from build123d import *

# Parameters (mm, degrees)
F0_W      = 50.8
F0_H      = 50.8
F0_W_2    = 39.37
F0_H_2    = 39.37
F1_DEPTH  = 25.4
F2_R      = 6.985
F3_DEPTH  = 50.801
F4_W      = 88.9
F4_H      = 279.4
F4_W_2    = 39.37
F4_H_2    = 39.37
F5_DEPTH  = 25.4
F6_W      = 76.2
F6_H      = 101.6
F7_DEPTH  = 3.175
F8_W      = 69.85
F8_H      = 101.6
F9_DEPTH  = 17.145
F10_W     = 69.85
F10_H     = 101.6
F11_DEPTH = 17.145
F12_W     = 38.1
F12_H     = 3.175
F13_DEPTH = 69.851
F15_DEPTH = 88.9


with BuildPart() as f1:
    # F0 (on Top) → F1 (new body)
    with BuildSketch(Plane.XY):
        Rectangle(F0_W, F0_H)
        Rectangle(F0_W_2, F0_H_2, mode=Mode.SUBTRACT)
    extrude(amount=F1_DEPTH)

    # F2 (on face) → F3 (cut, through all)
    with BuildSketch(Plane.XZ.offset(25.4)):
        with Locations((0, 12.7)):
            Circle(F2_R)
    extrude(amount=-F3_DEPTH, mode=Mode.SUBTRACT)

    # F4 (on face) → F5 (join)
    with BuildSketch(Plane.XY.offset(25.4)):
        Rectangle(F4_W, F4_H)
        Rectangle(F4_W_2, F4_H_2, mode=Mode.SUBTRACT)
    extrude(amount=F5_DEPTH)

    # F6 (on face) → F7 (cut)
    with BuildSketch(Plane(origin=(0, 0, 25.4), x_dir=(1, 0, 0), z_dir=(0, 0, -1))):
        with Locations((0, -82.55)):
            Rectangle(F6_W, F6_H)
        with Locations((0, 82.55)):
            Rectangle(F6_W, F6_H)
    extrude(amount=-F7_DEPTH, mode=Mode.SUBTRACT)

    # F8 (on face) → F9 (cut)
    with BuildSketch(Plane(origin=(0, 0, 28.575), x_dir=(1, 0, 0), z_dir=(0, 0, -1))):
        with Locations((0, -82.55)):
            Rectangle(F8_W, F8_H)
    extrude(amount=-F9_DEPTH, mode=Mode.SUBTRACT)

    # F10 (on face) → F11 (cut)
    with BuildSketch(Plane(origin=(0, 0, 28.575), x_dir=(1, 0, 0), z_dir=(0, 0, -1))):
        with Locations((0, 82.55)):
            Rectangle(F10_W, F10_H)
    extrude(amount=-F11_DEPTH, mode=Mode.SUBTRACT)

    # F12 (on face) → F13 (cut, through all)
    with BuildSketch(Plane.YZ.offset(25.4)):
        with Locations((0, 1.5875)):
            Rectangle(F12_W, F12_H)
    extrude(amount=-F13_DEPTH, mode=Mode.SUBTRACT)

    # F14 (on face) → F15 (join, through all)
    with BuildSketch(Plane.YZ.offset(44.45)):
        Polygon((-139.7, 25.4), (-139.7, 50.8), (-165.1, 50.8), align=None)
        Polygon((139.7, 50.8), (139.7, 25.4), (165.1, 50.8), align=None)
    extrude(amount=-F15_DEPTH)


solid = f1.part
Source: CAD feature listing. Evaluate the final solid. Frame: model axes, mm. A direction names the side the tool comes from. Round coordinates to 2 decimals unless told otherwise and drop trailing zeros. Write each loop counter-clockwise with the first axis right and the second up, starting at its lowest first coordinate (ties: lowest second). Pieces come first, ordered by that corner, then holes. Notation, with made-up numbers: M 77.25,53 L 134.25,53 A35 cw 134.25,85 Z; hole C -37.75,74.5 d7. An arc over 180 degrees is marked long. One line per item, written item: value. Start each with the question number.
Item 1: Section query D-D (x = 15.5). Return the cut outline in (y, z) (3 decimals).
Item 2: Set-up query: faces 4 (the flat face through (5, 25.4, 18)), 5 (the flat face through (-1, -31.75, 35)), 6 (the flat face through (25.4, 0, 13)), 7 (the flat face through (-19.685, 0, 31)), 8 (the flat face through (-44.45, -2, 38)). Return all of +Z, -Z, +X, -X, +Y, -Y with unobstructed straight access to the full face (end or side cutting, diameter ignored); none if empty.
Item 3: Ray query, L1, parallel to Y at x = -19, z = 7.5 (3 decimals); L2, parallel to Z at x = 0, y = -23.05 (3 decimals); L3, parallel to X at y = 22, z = 12. Return the intervals inside material, ascending. Write a range as from..to.
Item 4: Section query B-B (z = 12.7). Return the cut outline in (x, y) (3 decimals), plus the area to 3 significant figures.
Item 5: Mould query, pull axis Y, two halves, no side actions, for faces 1 (the flat face through (0.6, 152.2, 37.9)), 2 (the flat face through (23, 0, 3.175)), 3 (the flat face through (20, 2, 50.8)). Classes: pulls with the +Y half, pulls with the -Y half, needs draft (parallel to the pull), parting line crosses it, or undercut.
Item 6: Section query C-C (y = 81.5). Return the cut outline in (x, z) (3 decimals).
Item 7: Pin query (flat end, axial travel): pin 1 (7.5 mm diameter, centred on x = -11, z = 15.5, fed in from +Y); pin 2 (4 mm diameter, centred on x = -1, z = 28.5, fed in from +Y); pin 3 (3 mm diameter, centred on x = 23, y = 8.5, fed in from -Z) (3 decimals). Return the tip coordinate at first contact, or that it passes through.
Item 8: Section query A-A (z = 35). Return the cut outline in (x, y) (3 decimals).
Result set:
1. outline: M -165.1,50.8 L -139.7,25.4 L -133.35,25.4 L -133.35,45.72 L -31.75,45.72 L -31.75,25.4 L -25.4,25.4 L -25.4,0 L -19.685,0 L -19.685,50.8 Z; M 19.685,0 L 25.4,0 L 25.4,25.4 L 31.75,25.4 L 31.75,45.72 L 133.35,45.72 L 133.35,25.4 L 139.7,25.4 L 165.1,50.8 L 19.685,50.8 Z
2. face 4: -Z, +X, -X, +Y
2. face 5: -Z
2. face 6: -Z, +X, +Y, -Y
2. face 7: +Z, -Z
2. face 8: +Z, -Z, -X, +Y, -Y
3. L1: y = -25.4..-19.685, 19.685..25.4
3. L2: z = 0..5.715, 19.685..50.8
3. L3: x = -25.4..-6.95, 6.95..25.4
4. outline: M -25.4,-25.4 L -6.985,-25.4 L -6.985,-19.685 L -19.685,-19.685 L -19.685,19.685 L -6.985,19.685 L -6.985,25.4 L -25.4,25.4 Z; M 6.985,-25.4 L 25.4,-25.4 L 25.4,25.4 L 6.985,25.4 L 6.985,19.685 L 19.685,19.685 L 19.685,-19.685 L 6.985,-19.685 Z
4. area: 871 mm²
5. face 1: pulls with the +Y half
5. face 2: undercut
5. face 3: needs draft
6. outline: M -44.45,25.4 L -38.1,25.4 L -38.1,28.575 L -34.925,28.575 L -34.925,45.72 L 34.925,45.72 L 34.925,28.575 L 38.1,28.575 L 38.1,25.4 L 44.45,25.4 L 44.45,50.8 L -44.45,50.8 Z
7. pin 1: stops at y = 25.4
7. pin 2: stops at y = 144.8
7. pin 3: stops at z = 3.175
8. outline: M -44.45,-149.3 L 44.45,-149.3 L 44.45,149.3 L -44.45,149.3 Z; hole M -34.925,-133.35 L 34.925,-133.35 L 34.925,-31.75 L -34.925,-31.75 Z; hole M -34.925,31.75 L 34.925,31.75 L 34.925,133.35 L -34.925,133.35 Z; hole M -19.685,-19.685 L 19.685,-19.685 L 19.685,19.685 L -19.685,19.685 Z
